Verification items for this drawing (mm, ordinates from the low corner). Round coordinates to 2 decimals unless told otherwise and drop trailing zeros. Order: outer loops, then holes, each group sorted by start corner. A loop starts at its lowest first (then second) coordinate and runs counter-clockwise, first axis right, second up. Notation, with made-up numbers: (37.25, -12.5) -> (82.25, -12.5) arc R23 ccw to (82.25, 21.5) -> close; hole circle Ø8 at (-35, 45). An arc over 180 degrees is marked (long way). Answer in a Markdown table with one row per item. Add a question column.
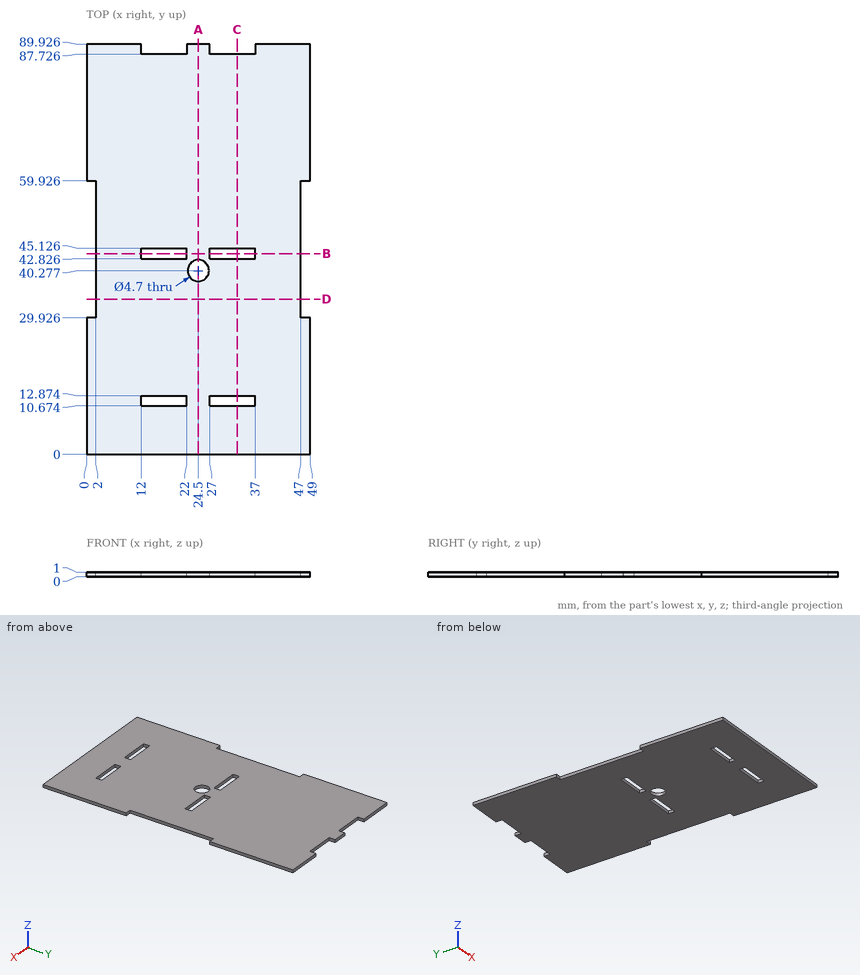
1) Cross-section at A-A, the plane x = 24.5. Record the boundary of the cut face in (y, z).
2) Cross-section at D-D, the plane y = 34. Record the boundary of the cut face in (x, z).
3) Cross-section at B-B, the plane y = 44. Record the boundary of the cut face in (x, z).
4) Depth check by flat-ended pin: P1, Ø0.5, axis at x = 30, z = 0.5, coming from the +Y side. Enter the tip coordinate at first touch or a pass-through.
5) Thickness scan on L1, parallel to Y at x = 16, z = 0.9; L2, parallel to X at y = 44.5, z = 0.85; L3, parallel to Y at x = 24.5, z = 0.6. Record the ranges inside material, lowest first. Write a range as [from, to].
6) Cross-section at C-C, the plane x = 33. Record the boundary of the cut face in (y, z).
Results below:
| question | item | result |
|---|---|---|
| 1 | outline | (0, 0) -> (37.93, 0) -> (37.93, 1) -> (0, 1) -> close; (42.63, 0) -> (89.93, 0) -> (89.93, 1) -> (42.63, 1) -> close |
| 2 | outline | (2, 0) -> (47, 0) -> (47, 1) -> (2, 1) -> close |
| 3 | outline | (2, 0) -> (12, 0) -> (12, 1) -> (2, 1) -> close; (22, 0) -> (27, 0) -> (27, 1) -> (22, 1) -> close; (37, 0) -> (47, 0) -> (47, 1) -> (37, 1) -> close |
| 4 | P1 | y = 87.73 |
| 5 | L1 | [0, 10.67], [12.87, 42.83], [45.13, 87.73] |
| 5 | L2 | [2, 12], [22, 27], [37, 47] |
| 5 | L3 | [0, 37.93], [42.63, 89.93] |
| 6 | outline | (0, 0) -> (10.67, 0) -> (10.67, 1) -> (0, 1) -> close; (12.87, 0) -> (42.83, 0) -> (42.83, 1) -> (12.87, 1) -> close; (45.13, 0) -> (87.73, 0) -> (87.73, 1) -> (45.13, 1) -> close |
